from build123d import *

# Parameters (mm, degrees)
SKETCH1_W                           = 65
SKETCH1_H                           = 150
SKETCH1_W_2                         = 55
SKETCH1_H_2                         = 140
BOSS_EXTRUDE1_DEPTH                 = 50
SKETCH2_R                           = 1.25
CUT_EXTRUDE1_DEPTH                  = 112.130553854
SKETCH3_R                           = 7.75
CUT_EXTRUDE2_DEPTH                  = 112.130553854
M3X0_5_TAPPED_HOLE3_D               = 2.5
M3X0_5_TAPPED_HOLE3_DEPTH           = 5
M3X0_5_TAPPED_HOLE3_TIP             = 0.751075774
M3X0_5_TAPPED_HOLE3_ON_FACE_2_D     = 2.5
M3X0_5_TAPPED_HOLE3_ON_FACE_2_DEPTH = 5
M3X0_5_TAPPED_HOLE3_ON_FACE_2_TIP   = 0.751075774
SKETCH10_W                          = 38
SKETCH10_H                          = 4
SKETCH10_R                          = 0.5
BOSS_EXTRUDE4_DEPTH                 = 10
M2X0_4_TAPPED_HOLE1_D               = 1.6
M2X0_4_TAPPED_HOLE1_DEPTH           = 10
M2X0_4_TAPPED_HOLE1_TIP             = 0.480688495
SKETCH4_R                           = 11
BOSS_EXTRUDE5_DEPTH                 = 10
SKETCH15_R                          = 1
BOSS_EXTRUDE6_DEPTH                 = 6.5


with BuildPart() as part:
    # Sketch1 → Boss-Extrude1 (new body)
    with BuildSketch(Plane(origin=(0, 0, 0), x_dir=(0, 1, 0), z_dir=(0, 0, 1))):
        Rectangle(SKETCH1_W, SKETCH1_H)
        Rectangle(SKETCH1_W_2, SKETCH1_H_2, mode=Mode.SUBTRACT)
    extrude(amount=BOSS_EXTRUDE1_DEPTH)

    # Sketch2 → Cut-Extrude1 (cut, through all)
    with BuildSketch(Plane.XZ.offset(32.5)):
        with Locations(Location((-60, 25, 0), (0, 0, 270))):
            Circle(SKETCH2_R)
        with Locations(Location((60, 25, 0), (0, 0, 270))):
            Circle(SKETCH2_R)
    extrude(amount=-CUT_EXTRUDE1_DEPTH, mode=Mode.SUBTRACT)

    # Sketch3 → Cut-Extrude2 (cut, through all)
    with BuildSketch(Plane.XZ.offset(32.5)):
        with Locations(Location((-36.75, 25, 0), (0, 0, 270))):
            Circle(SKETCH3_R)
    extrude(amount=-CUT_EXTRUDE2_DEPTH, mode=Mode.SUBTRACT)

    # M3x0.5 Tapped Hole3
    with Locations(Plane(origin=(-60, -32.5, 25), x_dir=(0, 0, -1), z_dir=(0, -1, 0))):
        with Locations((0, 0), (0, 120)):
            Hole(M3X0_5_TAPPED_HOLE3_D / 2, depth=M3X0_5_TAPPED_HOLE3_DEPTH)
            with Locations((0, 0, -(M3X0_5_TAPPED_HOLE3_DEPTH + M3X0_5_TAPPED_HOLE3_TIP / 2))):  # 118° drill point
                Cone(0, M3X0_5_TAPPED_HOLE3_D / 2, M3X0_5_TAPPED_HOLE3_TIP, mode=Mode.SUBTRACT)

    # M3x0.5 Tapped Hole3 on face 2
    with Locations(Plane(origin=(60, 32.5, 25), x_dir=(0, 0, -1), z_dir=(0, -1, 0))):
        with Locations((0, 0), (0, -120)):
            Hole(M3X0_5_TAPPED_HOLE3_ON_FACE_2_D / 2, depth=M3X0_5_TAPPED_HOLE3_ON_FACE_2_DEPTH)
            with Locations((0, 0, -(M3X0_5_TAPPED_HOLE3_ON_FACE_2_DEPTH + M3X0_5_TAPPED_HOLE3_ON_FACE_2_TIP / 2))):  # 118° drill point
                Cone(0, M3X0_5_TAPPED_HOLE3_ON_FACE_2_D / 2, M3X0_5_TAPPED_HOLE3_ON_FACE_2_TIP, mode=Mode.SUBTRACT)

    # Sketch10 → Boss-Extrude4 (add)
    # profile 1 of 2: a face of its own
    with BuildSketch(Plane(origin=(0, -27.5, 0), x_dir=(-1, 0, 0), z_dir=(0, 1, 0))):
        with Locations((24.25, 40)):
            Rectangle(SKETCH10_W, SKETCH10_H)
        with Locations(Location((7.25, 40, 0), (0, 0, 90))):
            Circle(SKETCH10_R, mode=Mode.SUBTRACT)
        with Locations(Location((41.25, 40, 0), (0, 0, 90))):
            Circle(SKETCH10_R, mode=Mode.SUBTRACT)
    # profile 2 of 2: a face of its own
    with BuildSketch(Plane(origin=(0, -27.5, 0), x_dir=(-1, 0, 0), z_dir=(0, 1, 0))):
        with Locations((24.25, 10)):
            Rectangle(SKETCH10_W, SKETCH10_H)
        with Locations(Location((7.25, 10, 0), (0, 0, 90))):
            Circle(SKETCH10_R, mode=Mode.SUBTRACT)
        with Locations(Location((41.25, 10, 0), (0, 0, 90))):
            Circle(SKETCH10_R, mode=Mode.SUBTRACT)
    extrude(amount=BOSS_EXTRUDE4_DEPTH)

    # M2x0.4 Tapped Hole1
    with Locations(Plane(origin=(-7.25, -17.5, 10), x_dir=(0, 0, 1), z_dir=(0, 1, 0))):
        with Locations((0, 0), (30, 0), (30, -34), (0, -34)):
            Hole(M2X0_4_TAPPED_HOLE1_D / 2, depth=M2X0_4_TAPPED_HOLE1_DEPTH)
            with Locations((0, 0, -(M2X0_4_TAPPED_HOLE1_DEPTH + M2X0_4_TAPPED_HOLE1_TIP / 2))):  # 118° drill point
                Cone(0, M2X0_4_TAPPED_HOLE1_D / 2, M2X0_4_TAPPED_HOLE1_TIP, mode=Mode.SUBTRACT)

    # Sketch4 → Boss-Extrude5 (add)
    with BuildSketch(Plane.YZ.offset(75)):
        with Locations(Location((0, 25, 0), (0, 0, 270))):
            Circle(SKETCH4_R)
    extrude(amount=BOSS_EXTRUDE5_DEPTH)

    # Sketch15 → Boss-Extrude6 (add)
    with BuildSketch(Plane.YZ.offset(85)):
        with Locations(Location((0, 33, 0), (0, 0, 90))):
            Circle(SKETCH15_R)
        with Locations(Location((8, 25, 0), (0, 0, 90))):
            Circle(SKETCH15_R)
        with Locations(Location((0, 17, 0), (0, 0, 90))):
            Circle(SKETCH15_R)
        with Locations(Location((-8, 25, 0), (0, 0, 90))):
            Circle(SKETCH15_R)
    extrude(amount=BOSS_EXTRUDE6_DEPTH)


solid = part.part
Model file for the job. Use its own axes, mm. A direction names the side the tool comes from. Give positions to 0.01 mm unless a question says otherwise; leave off trailing zeros. Order: outer loops, then holes, each group sorted by start corner. A loop starts at its lowest first (then second) coordinate and runs counter-clockwise, first axis right, second up. Notation, with made-up numbers: M 49,-18.75 L 81,-18.75 A36 ccw 81,15.25 Z; hole C 54.5,62 d1. An arc over 180 degrees is marked long. Put each result on its own line as item: value. Start each with the question number.
(1) Pin check, flat tips, straight feed: pin 1 Ø3 at (x, y) = (-17.5, -23.5) entering from -Z; pin 2 Ø2 at (y, z) = (-21.5, 11) entering from +X; pin 3 Ø2 at (x, z) = (-60, 25) entering from -Y; pin 4 Ø11 at (x, y) = (-18, -21.5) entering from +Z. Stop position of each tip, or through.
(2) Tool access for faces 1 (the face through (85, 0, 25)), 2 (the face through (-43.25, -23, 10)), 3 (the face through (-24, -23, 38)): list every direction of +Z, -Z, +X, -X, +Y, -Y with a clear straight run to the whole face (end or side of a thin tool).
(3) Band-saw the part on A-A on y = 12.5. Give the cut face in (x, z).
(4) Band-saw the part on B-B on x = -18. Give the cut face in (y, z), then the cut area to 3 significant figures.
(5) Drill centre lines: L1, parallel to X at y = -20, z = 40; L2, parallel to X at y = -28.5, z = 25; L3, parallel to Z at x = -7.25, y = -20. Where is each one in solid material? Low to high. Write a range as [from, to].
(6) Band-saw the part on D-D on y = -3. Give the cut face in (x, z), then the cut area to 3 significant figures.
(7) Band-saw the part on C-C on x = -64. Give the cut face in (y, z).
(8) Pull direction Y, two halves, no side cores. Call faces 4 (the face through (-24, -23, 42)), 5 (the face through (75, -0.5, 13.5)), 6 (the face through (79.93, -4.213, 14.839)): released by +Y, released by -Y, zero draft, split by the parting line, or undercut.
Results below:
1. pin 1: stops at z = 8
1. pin 2: stops at x = 75
1. pin 3: passes through
1. pin 4: stops at z = 42
2. face 1: +X
2. face 2: +Z, -Z
2. face 3: none
3. outline: M -75,0 L -70,0 L -70,50 L -75,50 Z; M 70,0 L 75,0 L 75,50 L 70,50 Z
4. outline: M -32.5,0 L -27.5,0 L -27.5,8 L -17.5,8 L -17.5,12 L -27.5,12 L -27.5,38 L -17.5,38 L -17.5,42 L -27.5,42 L -27.5,50 L -32.5,50 Z; M 27.5,0 L 32.5,0 L 32.5,50 L 27.5,50 Z
4. area: 580 mm2
5. L1: x = [-75, -70], [-43.25, -42.05], [-40.45, -8.05], [-6.45, -5.25], [70, 75]
5. L2: x = [-75, -61.25], [-58.75, -44.5], [-29, 58.75], [61.25, 75]
5. L3: z = [8, 9.2], [10.8, 12], [38, 39.2], [40.8, 42]
6. outline: M -75,0 L -70,0 L -70,50 L -75,50 Z; M 70,0 L 75,0 L 75,14.42 L 85,14.42 L 85,35.58 L 75,35.58 L 75,50 L 70,50 Z
6. area: 712 mm2
7. outline: M -32.5,0 L -27.5,0 L -27.5,50 L -32.5,50 Z; M 27.5,0 L 32.5,0 L 32.5,50 L 27.5,50 Z
8. face 4: undercut
8. face 5: zero draft
8. face 6: split by the parting line
